The listing builds one solid part. Answer for the finished solid, in the listing's coordinates (mm). A direction names the side the tool comes from. Round coordinates to 2 decimals unless told otherwise and drop trailing zeros. Order: outer loops, then holes, each group sorted by start corner. A loop starts at its lowest first (then second) coordinate and runs counter-clockwise, first axis right, second up. Notation, with made-up numbers: (10, 69.5) -> (69, 69.5) arc R32 ccw to (69, 101.5) -> close; hole circle Ø8 at (22.25, 2). An arc over 180 degrees is marked (long way). Answer in a Markdown table with one row per item. Add a question column.
```python
from build123d import *

# Parameters (mm, degrees)
BOSS_EXTRUDE1_DEPTH = 7
SKETCH3_R           = 1.7
CUT_EXTRUDE2_DEPTH  = 60


with BuildPart() as part:
    # Sketch1 → Boss-Extrude1 (new body)
    with BuildSketch(Plane(origin=(0, 0, 0), x_dir=(1, 0, 0), z_dir=(0, 1, 0))):
        Polygon((-87.25, -27.005178012), (-87.25, -44.605178012), (-54.181, -44.605178012), (-54.181, -27.005178012), (-46.181, -27.005178012), (-46.181, -49.605178012), (-64.006, -49.605178012), (-77.425, -49.605178012), (-95.25, -49.605178012), (-95.25, -27.005178012), align=None)
    extrude(amount=BOSS_EXTRUDE1_DEPTH)

    # Sketch3 → Cut-Extrude2 (cut)
    with BuildSketch(Plane(origin=(-46.181, 0, 0), x_dir=(0, 0, -1), z_dir=(1, 0, 0))):
        with Locations((-31.905178012, 3.5)):
            Circle(SKETCH3_R)
    extrude(amount=-CUT_EXTRUDE2_DEPTH, mode=Mode.SUBTRACT)


solid = part.part
```
1. The part is cut by section A-A (z = 41.5). Give the vertices of the cut face in (x, y), then the cut area to 3 significant figures.
2. For faces 5 (the flat face through (-50, 3, 27.005)), 6 (the flat face through (-87.25, 3, 36)), determine the directions among +Z, -Z, +X, -X, +Y, -Y from which every point of the face is accessible in a straight line to the end or side of a thin tool.
3. The mould has two halves that part along Z. Classify faces 1 (the flat face through (-65, 0, 46)), 2 (the cylindrical face through (-50.125, 2.849, 30.335)), 3 (the cylindrical face through (-91.194, 2.849, 30.335)), 4 (the flat face through (-91, 3, 27.005)): released by +Z, released by -Z, zero draft, split by the parting line, or undercut.
4. The part is cut by section C-C (z = 33). Give the vertices of the cut face in (x, y).
5. The part is cut by section B-B (y = 3.5). Give the vertices of the cut face in (x, z), then the cut area to 3 significant figures.
6. Each of these flat-tipped pins is pushed along its axis until it touches: pin 1 (2 mm diameter, centred on y = 3.5, z = 31.91, fed in from -X); pin 2 (2 mm diameter, centred on x = -69.5, y = 2, fed in from -Z). Where does it stop, or does it pass through?
7. Straight lines are drawn through the part: line 1 along X through (y, z) = (4.5, 33.5); line 2 along Z through (x, y) = (-61, 6.5). For each, find the intervals that lie inside material, in ascending order.
8. The part is cut by section D-D (x = -74). Give the vertices of the cut face in (y, z).
Report:
| question | item | result |
|---|---|---|
| 1 | outline | (-95.25, 0) -> (-87.25, 0) -> (-87.25, 7) -> (-95.25, 7) -> close; (-54.18, 0) -> (-46.18, 0) -> (-46.18, 7) -> (-54.18, 7) -> close |
| 1 | area | 112 mm^2 |
| 2 | face 5 | -Z, +X, -X, +Y, -Y |
| 2 | face 6 | -Z, +Y, -Y |
| 3 | face 1 | zero draft |
| 3 | face 2 | undercut |
| 3 | face 3 | undercut |
| 3 | face 4 | released by -Z |
| 4 | outline | (-95.25, 0) -> (-87.25, 0) -> (-87.25, 2.2) -> (-95.25, 2.2) -> close; (-95.25, 4.8) -> (-87.25, 4.8) -> (-87.25, 7) -> (-95.25, 7) -> close; (-54.18, 0) -> (-46.18, 0) -> (-46.18, 2.2) -> (-54.18, 2.2) -> close; (-54.18, 4.8) -> (-46.18, 4.8) -> (-46.18, 7) -> (-54.18, 7) -> close |
| 5 | outline | (-95.25, 27.01) -> (-87.25, 27.01) -> (-87.25, 30.21) -> (-95.25, 30.21) -> close; (-95.25, 33.61) -> (-87.25, 33.61) -> (-87.25, 44.61) -> (-54.18, 44.61) -> (-54.18, 33.61) -> (-46.18, 33.61) -> (-46.18, 49.61) -> (-95.25, 49.61) -> close; (-54.18, 27.01) -> (-46.18, 27.01) -> (-46.18, 30.21) -> (-54.18, 30.21) -> close |
| 5 | area | 473 mm^2 |
| 6 | pin 1 | passes through |
| 6 | pin 2 | stops at z = 44.61 |
| 7 | line 1 | x = -95.25 to -87.25, -54.18 to -46.18 |
| 7 | line 2 | z = 44.61 to 49.61 |
| 8 | outline | (0, 44.61) -> (7, 44.61) -> (7, 49.61) -> (0, 49.61) -> close |
